Build history of the part. All positions in model axes, mm. Face numbers are marked on the shaded views. A direction names the side the tool comes from. Round coordinates to 2 decimals unless told otherwise and drop trailing zeros. Order: outer loops, then holes, each group sorted by start corner. A loop starts at its lowest first (then second) coordinate and runs counter-clockwise, first axis right, second up. Notation, with made-up numbers: (15.25, 71) -> (26.25, 71) arc R30 ccw to (26.25, 105) -> close; hole circle Ø8 at (-7.75, -6). An arc over 180 degrees is marked (long way). Use a Markdown table: item, result. Add a question column.
Item 1: Pin check, flat tips, straight feed: pin 1 (1.5 mm diameter, centred on x = 1, z = -3, fed in from +Y); pin 2 (1 mm diameter, centred on y = 1, z = -2.5, fed in from +X); pin 3 (1.5 mm diameter, centred on x = 2, z = -0.5, fed in from +Y). Stop position of each tip, or through.
Item 2: Slice it at A-A, the plane x = 0. Give the cut face in (y, z), plus the area to 3 significant figures.
Item 3: Probe L1, parallel to Z at x = 0, y = 1; L2, parallel to Y at x = 0.25, z = 3.25; L3, parallel to X at y = 0.5, z = 1.5. List the from-to ranges inside material, lowest first.
Item 4: 3-axis set-ups, long thin cutter, end or side, ignore diameter. For the marked faces 4, 5 and 6: which of +Z, -Z, +X, -X, +Y, -Y reach the whole face in a straight line?
Item 5: Slice it at D-D, the plane y = 5.5. Give the cut face in (x, z), plus the area to 3 significant figures.
Item 6: Slice it at C-C, the plane y = 2.5. Give the cut face in (x, z).
Item 7: Slice it at B-B, the plane z = -1. Give the cut face in (x, y), plus the area to 3 significant figures.
Item 8: Two-plate mould, pull along X, no slides. Class the marked faces 1, 2 and 3: released by +X, released by -X, zero draft, split by the parting line, or undercut.
from build123d import *

# Parameters (mm, degrees)
BOSS_EXTRUDE1_DEPTH = 3.4
SKETCH4_R           = 2.5
CUT_EXTRUDE1_DEPTH  = 1.2


with BuildPart() as part:
    # Sketch1 → Boss-Extrude1 (new body)
    with BuildSketch(Plane(origin=(0, 0, 0), x_dir=(1, 0, 0), z_dir=(0, 1, 0))):
        Polygon((2.25, 3.897114317), (-2.25, 3.897114317), (-4.5, 0), (-2.25, -3.897114317), (2.25, -3.897114317), (4.5, 0), align=None)
    extrude(amount=BOSS_EXTRUDE1_DEPTH)

    # Sketch2 → Revolve1 (revolve)
    with BuildSketch(Plane(origin=(0, 3.4, 0), x_dir=(1, 0, 0), z_dir=(0, 1, 0))):
        with BuildLine():
            Line((0, 3), (0, -3))
            ThreePointArc((0, -3), (3, 0), (0, 3))
        make_face()
    revolve(axis=Axis((0, 3.4, -3), (0, 0, 1)))

    # Sketch4 → Cut-Extrude1 (cut)
    with BuildSketch(Plane.XZ):
        Circle(SKETCH4_R)
    extrude(amount=-CUT_EXTRUDE1_DEPTH, mode=Mode.SUBTRACT)


solid = part.part
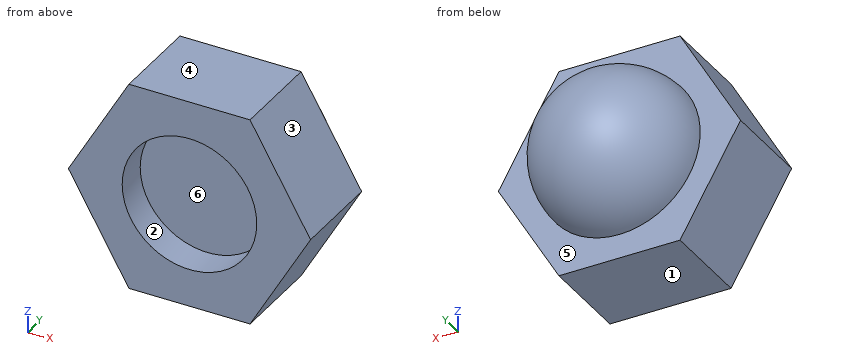
Check sheet entries:
| question | item | result |
|---|---|---|
| 1 | pin 1 | y = 5.18 |
| 1 | pin 2 | x = 3.35 |
| 1 | pin 3 | y = 6.1 |
| 2 | outline | (0, -3.9) -> (3.4, -3.9) -> (3.4, -3) arc R3 ccw to (3.4, 3) -> (3.4, 3.9) -> (0, 3.9) -> (0, 2.5) -> (1.2, 2.5) -> (1.2, -2.5) -> (0, -2.5) -> close |
| 2 | area | 34.6 mm2 |
| 3 | L1 | -3.9 to -2.5, 2.5 to 3.9 |
| 3 | L2 | 0 to 3.4 |
| 3 | L3 | -3.63 to -2, 2 to 3.63 |
| 4 | face 4 | +Z, +X, -X, +Y, -Y |
| 4 | face 5 | +Y |
| 4 | face 6 | -Y |
| 5 | outline | circle Ø4.28 at (0, 0) |
| 5 | area | 14.4 mm2 |
| 6 | outline | (-4.5, 0) -> (-2.25, -3.9) -> (2.25, -3.9) -> (4.5, 0) -> (2.25, 3.9) -> (-2.25, 3.9) -> close |
| 7 | outline | (-3.92, 0) -> (-2.29, 0) -> (-2.29, 1.2) -> (2.29, 1.2) -> (2.29, 0) -> (3.92, 0) -> (3.92, 3.4) -> (2.83, 3.4) arc R2.83 ccw to (-2.83, 3.4) -> (-3.92, 3.4) -> close |
| 7 | area | 33.7 mm2 |
| 8 | face 1 | zero draft |
| 8 | face 2 | undercut |
| 8 | face 3 | released by +X |
